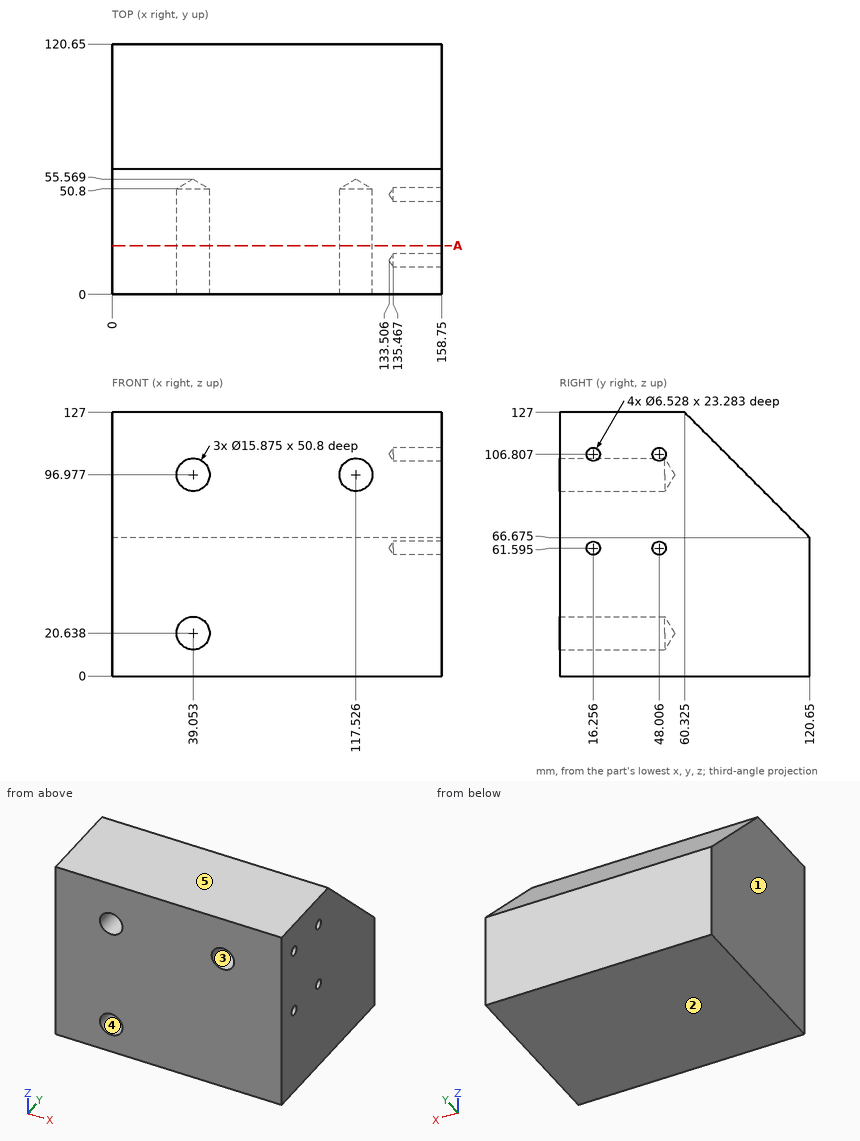
Geometry check sheet. Reference: drawing and pictorial views, mm from the part's lowest x, y, z. A direction names the side the tool comes from. Round coordinates to 2 decimals unless told otherwise and drop trailing zeros. Answer as CSV lines item,"result". Start each with the question number.
1) Material ranges on line 1 (Z direction, x = 46, y = 17) (1 decimal); line 2 (Z direction, x = 46, y = 88) (1 decimal); line 3 (Y direction, x = 64.5, z = 100) (1 decimal), recorded low to high. Write a range as from..to.
2) Tool access check on the marked faces 4 and 5. Record the directions out of +Z, -Z, +X, -X, +Y, -Y that give a thin tool (end or side, any length) a straight path to the whole face; none if there is none.
3) Go/stop test with flat-tipped pins: P1, Ø5, axis at y = 16.256, z = 61.595, coming from the +X side; P2, Ø4, axis at x = 128.5, y = 72, coming from the +Z side (1 decimal); P3, Ø12.5, axis at x = 39.05, z = 96.98, coming from the -Y side. Record where each tip stops, or that it passes through.
4) Section check A-A on y = 23.5. State how many separate pieces and enclosed holes the cut face has, and give its area (3 significant figures).
5) Release check for a two-part mould opening along Z. For the marked faces 1, 2 and 3 record: pulls with the +Z half, pulls with the -Z half, needs draft (parallel to the pull), parting line crosses it, or undercut.
Found:
1,line 1,"z = 0..16.8, 24.5..93.1, 100.8..127"
1,line 2,"z = 0..99.3"
1,line 3,"y = 0..87.3"
2,face 4,"-Y"
2,face 5,"+Z, +X, -X, +Y, -Y"
3,P1,"stops at x = 135.01"
3,P2,"stops at z = 117.3"
3,P3,"stops at y = 51.81"
4,separate pieces,"1"
4,enclosed holes,"3"
4,area,"19,600 mm^2"
5,face 1,"needs draft"
5,face 2,"pulls with the -Z half"
5,face 3,"undercut"
